Autodesk Inventor part; units mm, degrees
ref_plane "YZ Plane" through (0, 0, 0) normal (1, 0, 0) x (0, 1, 0)
ref_plane "XZ Plane" through (0, 0, 0) normal (0, 1, 0) x (-1, 0, 0)
ref_plane "XY Plane" through (0, 0, 0) normal (0, 0, 1) x (1, 0, 0)
sketch "Эскиз1" plane through (0, 2, -127) normal (0, 1, 0) x (1, 0, 0)
  circle A0 centre (-90.3481, -100.1076) radius 1.5
  circle A1 centre (90.3481, -153.8924) radius 1.5
  circle A2 centre (-90.3481, -153.8924) radius 1.5
  circle A3 centre (90.3481, -100.1076) radius 1.5
  circle A4 centre (51.0265, -155.3991) radius 1.5
  circle A5 centre (-67.0849, -171.4575) radius 1.5
  circle A6 centre (-44.4575, -59.9151) radius 1.5
  circle A7 centre (51.0265, -98.6009) radius 1.5
  circle A8 centre (28.3991, -75.9735) radius 1.5
  circle A9 centre (-67.0849, -82.5425) radius 1.5
  circle A10 centre (-28.3991, -178.0265) radius 1.5
  circle A11 centre (28.3991, -178.0265) radius 1.5
  circle A12 centre (67.0849, -171.4575) radius 1.5
  circle A13 centre (-51.0265, -155.3991) radius 1.5
  circle A14 centre (-28.3991, -75.9735) radius 1.5
  circle A15 centre (67.0849, -82.5425) radius 1.5
  circle A16 centre (44.4575, -59.9151) radius 1.5
  circle A17 centre (-51.0265, -98.6009) radius 1.5
  circle A18 centre (-44.4575, -194.0849) radius 1.5
  circle A19 centre (44.4575, -194.0849) radius 1.5
  arc A20 (-36.9892, -29.8002) -> (36.9892, -29.8002) centre (0, 0) ccw
  arc A21 (-36.9892, -29.8002) -> (-48.2758, -34.8835) centre (0, -127) ccw
  line L0 (-48.2758, -34.8835) -> (-38.4471, -44.7123)
  line L1 (-38.4471, -44.7123) -> (-82.2877, -88.5529)
  line L2 (-82.2877, -88.5529) -> (-92.1165, -78.7242)
  arc A22 (-92.1165, -78.7242) -> (-92.1165, -175.2758) centre (0, -127) ccw
  line L3 (-92.1165, -175.2758) -> (-82.2877, -165.4471)
  line L4 (-82.2877, -165.4471) -> (-38.4471, -209.2877)
  line L5 (-38.4471, -209.2877) -> (-48.2758, -219.1165)
  arc A23 (-48.2758, -219.1165) -> (-36.9892, -224.1998) centre (0, -127) ccw
  arc A24 (36.9892, -224.1998) -> (-36.9892, -224.1998) centre (0, -254) ccw
  arc A25 (36.9892, -224.1998) -> (48.2758, -219.1165) centre (0, -127) ccw
  line L6 (48.2758, -219.1165) -> (38.4471, -209.2877)
  line L7 (38.4471, -209.2877) -> (82.2877, -165.4471)
  line L8 (82.2877, -165.4471) -> (92.1165, -175.2758)
  arc A26 (92.1165, -175.2758) -> (92.1165, -78.7242) centre (0, -127) ccw
  line L9 (92.1165, -78.7242) -> (82.2877, -88.5529)
  line L10 (82.2877, -88.5529) -> (38.4471, -44.7123)
  line L11 (38.4471, -44.7123) -> (48.2758, -34.8835)
  arc A27 (48.2758, -34.8835) -> (36.9892, -29.8002) centre (0, -127) ccw
  line L12 (-67.0849, -82.5425) -> (-51.0265, -98.6009) construction
  circle A28 centre (0, -127) radius 69.3873
  line L13 (-62.0891, -96.0236) -> (-51.0265, -107.0862)
  line L14 (-51.0265, -107.0862) -> (-19.9138, -75.9735)
  line L15 (-19.9138, -75.9735) -> (-30.9764, -64.9109)
  line L16 (-51.0265, -146.9138) -> (-62.0891, -157.9764)
  line L17 (-19.9138, -178.0265) -> (-51.0265, -146.9138)
  line L18 (-30.9764, -189.0891) -> (-19.9138, -178.0265)
  line L19 (19.9138, -178.0265) -> (30.9764, -189.0891)
  line L20 (51.0265, -146.9138) -> (19.9138, -178.0265)
  line L21 (62.0891, -157.9764) -> (51.0265, -146.9138)
  line L22 (51.0265, -107.0862) -> (62.0891, -96.0236)
  line L23 (19.9138, -75.9735) -> (51.0265, -107.0862)
  line L24 (30.9764, -64.9109) -> (19.9138, -75.9735)
  point P0 (-59.0557, -90.5717)
sketch "Эскиз2_1" plane through (0, 2, 127) normal (0, 1, 0) x (1, 0, 0)
  circle A0 centre (0, 127) radius 104
  line L0 (-92.1165, 78.7242) -> (-82.2877, 88.5529)
  line L1 (-82.2877, 88.5529) -> (-38.4471, 44.7123)
  line L2 (-38.4471, 44.7123) -> (-48.2758, 34.8835)
  line L3 (48.2758, 34.8835) -> (38.4471, 44.7123)
  line L4 (38.4471, 44.7123) -> (82.2877, 88.5529)
  line L5 (82.2877, 88.5529) -> (92.1165, 78.7242)
  line L6 (82.2877, 165.4471) -> (38.4471, 209.2877)
  line L7 (38.4471, 209.2877) -> (48.2758, 219.1165)
  line L8 (92.1165, 175.2758) -> (82.2877, 165.4471)
  line L9 (-48.2758, 219.1165) -> (-38.4471, 209.2877)
  line L10 (-38.4471, 209.2877) -> (-82.2877, 165.4471)
  line L11 (-82.2877, 165.4471) -> (-92.1165, 175.2758)
sketch "Эскиз3" plane through (0, 2, 127) normal (0, 1, 0) x (1, 0, 0)
  circle A0 centre (-23.8556, 50.0189) radius 1.5
  circle A1 centre (23.8556, 50.0189) radius 1.5
  circle A2 centre (-23.8556, 203.9811) radius 1.5
  circle A3 centre (23.8556, 203.9811) radius 1.5
  point P0 (0, 127)
sketch "Эскиз6" plane through (0, 0, 0) normal (0, 1, 0) x (-1, 0, 0)
  circle A0 centre (0, 0) radius 49.5
  circle A1 centre (0, 0) radius 41
  dimension "d1" = 99
  dimension "d2" = 82
sketch "Эскиз7" plane through (0, 0, 0) normal (0, 1, 0) x (-1, 0, 0)
  circle A0 centre (90.3481, 26.8924) radius 1.5
  circle A1 centre (90.3481, -26.8924) radius 1.5
  circle A2 centre (23.8556, 76.9811) radius 1.5
  circle A3 centre (23.8556, -76.9811) radius 1.5
  circle A4 centre (-23.8556, -76.9811) radius 1.5
  circle A5 centre (-23.8556, 76.9811) radius 1.5
  circle A6 centre (-90.3481, 26.8924) radius 1.5
  circle A7 centre (-90.3481, -26.8924) radius 1.5
  circle A8 centre (0, 0) radius 28
  circle A9 centre (90.3481, 26.8924) radius 3.5
  circle A10 centre (90.3481, -26.8924) radius 3.5
  circle A11 centre (23.8556, -76.9811) radius 3.5
  circle A12 centre (-23.8556, -76.9811) radius 3.5
  circle A13 centre (-90.3481, -26.8924) radius 3.5
  circle A14 centre (-90.3481, 26.8924) radius 3.5
  circle A15 centre (23.8556, 76.9811) radius 3.5
  circle A16 centre (-23.8556, 76.9811) radius 3.5
  line L0 (0, 0) -> (28, 0) construction
  line L1 (23.8556, 76.9811) -> (27.3556, 76.9811) construction
  line L2 (90.3481, 26.8924) -> (90.3481, 30.3924) construction
  arc A17 (27.3556, 76.9811) -> (90.3481, 30.3924) centre (76.0802, 76.9811) ccw
  line L3 (27.3556, 76.9811) -> (27.3556, 30.3924) construction
  line L4 (27.3556, 30.3924) -> (90.3481, 30.3924) construction
  arc A18 (90.3481, -30.3924) -> (27.3556, -76.9811) centre (76.0802, -76.9811) ccw
  line L5 (0, 0) -> (0, 28) construction
  arc A19 (-90.3481, 30.3924) -> (-27.3556, 76.9811) centre (-76.0802, 76.9811) ccw
  arc A20 (-27.3556, -76.9811) -> (-90.3481, -30.3924) centre (-76.0802, -76.9811) ccw
  line L6 (90.3481, 26.8924) -> (93.8481, 26.8924) construction
  line L7 (90.3481, -26.8924) -> (93.8481, -26.8924) construction
  arc A21 (93.8481, 26.8924) -> (93.8481, -26.8924) centre (195.4124, 0) ccw
  arc A22 (-93.8481, -26.8924) -> (-93.8481, 26.8924) centre (-195.4124, 0) ccw
  line L8 (-23.8556, 76.9811) -> (-23.8556, 80.4811) construction
  line L9 (23.8556, 76.9811) -> (23.8556, 80.4811) construction
  arc A23 (-23.8556, 80.4811) -> (23.8556, 80.4811) centre (0, 160.0297) ccw
  arc A24 (23.8556, -80.4811) -> (-23.8556, -80.4811) centre (0, -160.0297) ccw
  point P0 (-27.3556, 76.9811)
  point P1 (-90.3481, 30.3924)
  point P2 (-93.8481, 26.8924)
  point P3 (-93.8481, -26.8924)
  point P4 (-90.3481, -30.3924)
  point P5 (-27.3556, -76.9811)
  point P6 (-23.8556, -80.4811)
  point P7 (23.8556, -80.4811)
  point P8 (90.3481, -30.3924)
  dimension "d3" = 56
  dimension "d4" = 7
extrude "Выдавливание1" add sketch "Эскиз7" along normal blind 2 contours A21 A9 A17 | A21 A10 A18 A11 A24 A12 A20 A13 A22 A14 A19 A16 A23 A15 A17 A9 | A21 A10 A18 | A15 A23 | A11 A24 | A16 A23 | A24 A12 | A14 A22 A19 | A20 A13 A22 picked at (26.6398, 76.5793) picked at (26.6398, -76.5793) picked at (-21.0707, 76.5822) picked at (-26.5069, -76.0401)
properties part number "dribler_floor"
Geometry check sheet. Reference: the model listing, model coordinates, mm. Coordinates: 2 decimals unless noted, no trailing zeros. Loops run counter-clockwise (first coordinate to the right, second up) from the corner with the lowest first, then second, coordinate; pieces in that order, holes last. Notation, with made-up numbers: (41, -40) -> (89, -40) arc R23 cw to (89, -31) -> close; hole circle Ø10 at (-7, -27.5). An arc over 180 degrees is marked (long way). Put each result on its own line as item: value.
1) Cross-section at A-A on z = 0. Record the boundary of the cut face in (x, y).
Result set:
outline: (-90.35, 0) -> (-28, 0) -> (-28, 2) -> (-90.35, 2) -> close; (28, 0) -> (90.35, 0) -> (90.35, 2) -> (28, 2) -> close
2) Cross-section at D-D on x = 38.5. Record the boundary of the cut face in (y, z).
Result set:
outline: (0, -45.97) -> (2, -45.97) -> (2, 45.97) -> (0, 45.97) -> close
3) Release check for a two-part mould opening along X. For faces 1 (the cylindrical face through (-25.865, 0.986, 10.724)), 2 (the flat face through (22, 0, 19)) record: released by +X, released by -X, zero draft, split by the parting line, or undercut.
Result set:
face 1: undercut
face 2: zero draft
4) Cross-section at C-C on y = 1.65. Count the separate pieces of the cut face and the enclosed holes in it, plus the area to 3 significant figures.
Result set:
separate pieces: 1
enclosed holes: 9
area: 15,400 mm^2
5) Cross-section at B-B on x = 0. Record the boundary of the cut face in (y, z).
Result set:
outline: (0, -76.98) -> (2, -76.98) -> (2, -28) -> (0, -28) -> close; (0, 28) -> (2, 28) -> (2, 76.98) -> (0, 76.98) -> close
6) Thickness scan on line 1 (X direction, y = 1.55, z = 67); line 2 (X direction, y = 0.1, z = 12); line 3 (Z direction, x = 0, y = 0.2). Record the ranges inside material, lowest first.
Result set:
line 1: x = -28.39 to 28.39
line 2: x = -91.04 to -25.3, 25.3 to 91.04
line 3: z = -76.98 to -28, 28 to 76.98
7) Gauge pin test, flat end, axial feed: pin 1 Ø1 at (x, y) = (-37, 1) entering from -Z. Record the tip position at first contact, or that the pin passes through.
Result set:
pin 1: stops at z = -48.56
